Answer from the drawing. Dimensions are ordinates in mm from the lowest x, y and z of the part. A direction names the side the tool comes from. Round coordinates to 2 decimals unless told otherwise and drop trailing zeros. Order: outer loops, then holes, each group sorted by start corner. A loop starts at its lowest first (then second) coordinate and runs counter-clockwise, first axis right, second up.
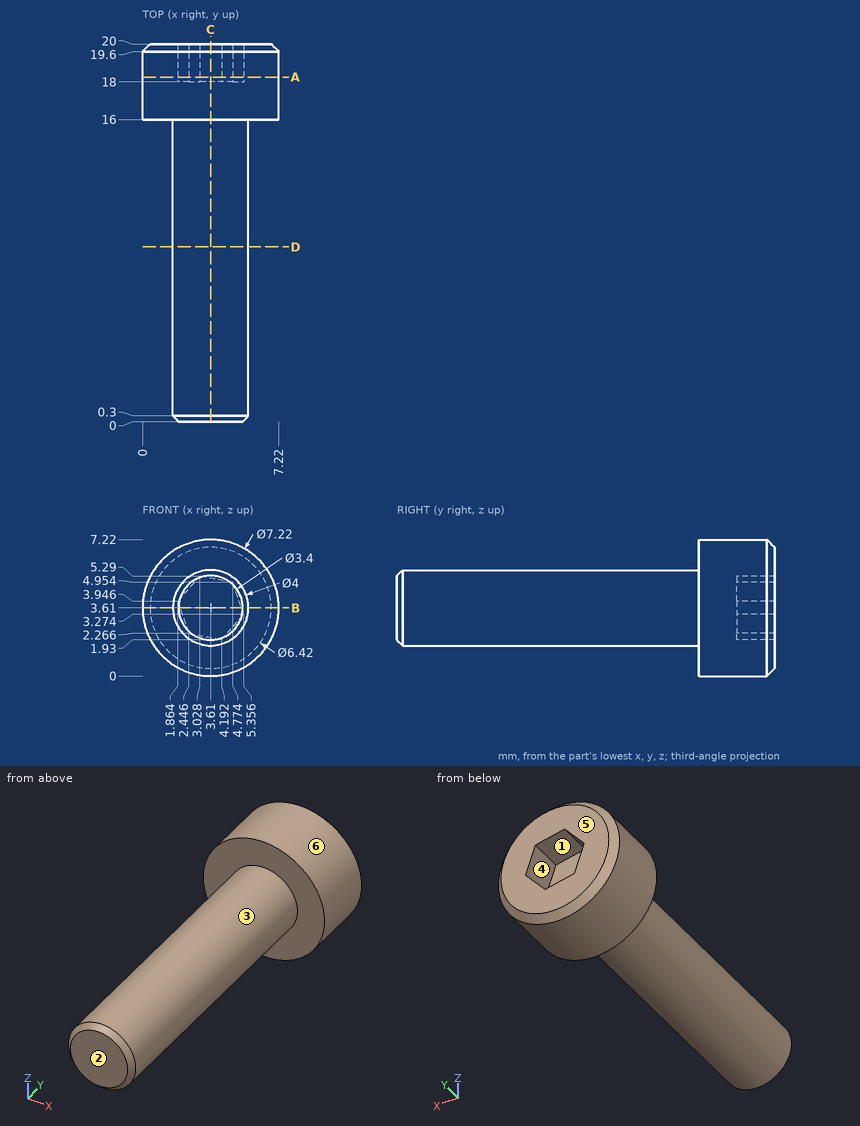
Q1. Straight lines are drawn through the part: probe 1 along Y at (x, z) = (1, 2.25); probe 2 along Y at (x, z) = (3, 3.5); probe 3 along Z at (x, y) = (3.5, 2.25). For each, find the intervals that lie inside material, in ascending order.
Outcome:
probe 1: y = 16 to 20
probe 2: y = 0 to 18
probe 3: z = 1.61 to 5.61
Q2. For the marked faces 1, 2 and 3, determine the directions among +Z, -Z, +X, -X, +Y, -Y from which every point of the face is accessible in a straight line to the end or side of a thin tool.
Outcome:
face 1: +Y
face 2: +Z, -Z, +X, -X, -Y
face 3: -Y
Q3. A cutting plane is placed at C-C, the plane x = 3.61. Give the vertices of the cut face in (y, z).
Outcome:
outline: (0, 1.91) - (0.3, 1.61) - (16, 1.61) - (16, 0) - (19.6, 0) - (20, 0.4) - (20, 2.04) - (18, 2.04) - (18, 5.18) - (20, 5.18) - (20, 6.82) - (19.6, 7.22) - (16, 7.22) - (16, 5.61) - (0.3, 5.61) - (0, 5.31) - close
Q4. For a pull along X with two mould halves and no side action, classify the marked faces 4, 5 and 6 as released by +X, released by -X, zero draft, split by the parting line, or undercut.
Outcome:
face 4: undercut
face 5: zero draft
face 6: split by the parting line
Q5. A cutting plane is placed at A-A, the plane y = 18.25. Give the vertices of the cut face in (x, z), plus the area to 3 significant figures.
Outcome:
outline: circle Ø7.22 at (3.61, 3.61); hole (1.86, 3.95) - (2.45, 2.27) - (4.19, 1.93) - (5.36, 3.27) - (4.77, 4.95) - (3.03, 5.29) - close
area: 32.7 mm2
Q6. A cutting plane is placed at B-B, the plane z = 3.61. Give the vertices of the cut face in (x, y).
Outcome:
outline: (0, 16) - (1.61, 16) - (1.61, 0.3) - (1.91, 0) - (5.31, 0) - (5.61, 0.3) - (5.61, 16) - (7.22, 16) - (7.22, 19.6) - (6.82, 20) - (5.24, 20) - (5.24, 18) - (1.98, 18) - (1.98, 20) - (0.4, 20) - (0, 19.6) - close
Q7. A cutting plane is placed at D-D, the plane y = 9.25. Give the vertices of the cut face in (x, z).
Outcome:
outline: circle Ø4 at (3.61, 3.61)
Q8. Flat-ended cylindrical pins translate along their axes: pin 1 (3 mm diameter, centred on y = 14, z = 1.5, fed in from -X) (1 decimal); pin 2 (2 mm diameter, centred on x = 5, y = 17.5, fed in from +Z); pin 3 (1 mm diameter, centred on x = 3.5, z = 4.5, fed in from +Y). Find the tip coordinate at first contact, or state that the pin passes through.
Outcome:
pin 1: stops at x = 1.7
pin 2: stops at z = 7.2
pin 3: stops at y = 18
